Input: part model. Units: mm. Frame: model coordinates. A direction names the side the tool comes from. Round coordinates to 2 decimals unless told otherwise and drop trailing zeros. Loops run counter-clockwise (first coordinate to the right, second up) from the corner with the lowest first, then second, coordinate; pieces in that order, holes last. Notation, with made-up numbers: (57.25, -35) -> (102.25, -35) arc R19 cw to (102.25, -31) -> close; hole circle Ø4 at (56, -15.5). An arc over 180 degrees is marked (long way). Answer in a Markdown table with one row per item. Add a question column.
Q1. Section A-A, the plane z = 61. Output: boundary loops of the cut face in (x, y), and give its area (3 significant figures).
Q2. Section D-D, the plane x = -3. Output: boundary loops of the cut face in (y, z).
Q3. Section C-C, the plane x = -71.5. Output: boundary loops of the cut face in (y, z), and give its area (3 significant figures).
Q4. Ray query, L1, parallel to X at y = 23, z = -43; L2, parallel to X at y = 9, z = 58; L3, parallel to Z at x = 46, y = 36. Return the intervals inside material, ascending. Write a range as from..to.
Q5. Mould query, pull axis X, two halves, no side actions, for faces 1 (the face through (1, 40, -41)), 2 (the face through (-25, 20, -140)), 3 (the face through (-18.714, 20, 69)). Classes: pulls with the +X half, pulls with the -X half, needs draft (parallel to the pull), parting line crosses it, or undercut.
Q6. Reachability of faces 4 (the face through (-76, 20, 20)), 5 (the face through (45.714, 20, 41)), 6 (the face through (76, 20, 20)), 7 (the face through (56, 20, -120)) from +Z, -Z, +X, -X, +Y, -Y: full face, straight path, thin tool, end or side. Return the list, or none.
Q7. Pin query (flat end, axial travel): pin 1 (10 mm diameter, centred on y = 36, z = 23, fed in from +X); pin 2 (12 mm diameter, centred on y = 11.5, z = -133.5, fed in from -X); pin 3 (12 mm diameter, centred on y = 19.5, z = 86.5, fed in from -X); pin 4 (10 mm diameter, centred on x = 56.5, y = 18, fed in from +Z). Return the tip coordinate at first contact, or that it passes through.
Q8. Section B-B, the plane y = 10.5. Output: boundary loops of the cut face in (x, z), and give its area (3 significant figures).
Autodesk Inventor part; units mm, degrees
ref_plane "YZ Plane" through (0, 0, 0) normal (1, 0, 0) x (0, 1, 0)
ref_plane "XZ Plane" through (0, 0, 0) normal (0, 1, 0) x (-1, 0, 0)
ref_plane "XY Plane" through (0, 0, 0) normal (0, 0, 1) x (1, 0, 0)
sketch "スケッチ1" plane through (0, 0, 0) normal (0, 1, 0) x (-1, 0, 0)
  line L0 (45.7143, 140) -> (25.7143, 140)
  line L1 (25.7143, 140) -> (25.7143, 0)
  line L2 (25.7143, 0) -> (45.7143, 0)
  line L3 (45.7143, 0) -> (45.7143, 140)
  line L4 (45.7143, 0) -> (0, 0)
  line L5 (0, 0) -> (0, -120)
  line L6 (0, -120) -> (45.7143, -120)
  line L7 (45.7143, -120) -> (45.7143, 0)
  line L8 (25, -120) -> (0, -120)
  line L9 (0, -120) -> (0, -160)
  line L10 (0, -160) -> (25, -160)
  line L11 (25, -160) -> (25, -120)
  line L12 (45.7143, -120) -> (65.7143, -120)
  line L13 (65.7143, -120) -> (65.7143, -60)
  line L14 (65.7143, -60) -> (45.7143, -60)
  line L15 (45.7143, -60) -> (45.7143, -120)
  line L16 (65.7143, -120) -> (85.7143, -120)
  line L17 (85.7143, -120) -> (85.7143, 20)
  line L18 (85.7143, 20) -> (65.7143, 20)
  line L19 (65.7143, 20) -> (65.7143, -120)
  line L20 (0, -220) -> (0, 200)
  line L21 (102.8571, 0) -> (-17.1429, 0)
  line L22 (25.7143, 0) -> (25.7143, 140)
  line L23 (25.7143, 0) -> (18.7143, 0)
  line L24 (18.7143, 0) -> (18.7143, 140)
  line L25 (18.7143, 140) -> (25.7143, 140)
  line L26 (25.7143, 140) -> (25.7143, 0)
  point P0 (0, 0)
  point P1 (65.7143, 0)
  point P2 (25.7143, 0)
  point P3 (18.7143, 0)
  dimension "d0" = 40
  dimension "d2" = 300
  dimension "d3" = 140
  dimension "d4" = 85.7143
  dimension "d5" = 20
  dimension "d6" = 20
  dimension "d7" = 25
  dimension "d10" = 60
  dimension "d11" = 7
extrude "押し出し1" add sketch "スケッチ1" along normal blind 40 contours L3 L2 L1 L0 | L1 L4 L24 L25 | L7 L6 L5 L4 L2 | L14 L13 L12 L7 | L21 L17 L16 L13 L19 | L19 L18 L17 L21 | L11 L10 L9 L6
mirror "ミラー1" about plane through (0, 0, 0) normal (1, 0, 0)
properties part number "human_model"
Answer block:
| question | item | result |
|---|---|---|
| 1 | outline | (-45.71, 0) -> (-18.71, 0) -> (-18.71, 40) -> (-45.71, 40) -> close; (18.71, 0) -> (45.71, 0) -> (45.71, 40) -> (18.71, 40) -> close |
| 1 | area | 2,160 mm^2 |
| 2 | outline | (0, -160) -> (40, -160) -> (40, 0) -> (0, 0) -> close |
| 3 | outline | (0, -120) -> (40, -120) -> (40, 20) -> (0, 20) -> close |
| 3 | area | 5,600 mm^2 |
| 4 | L1 | -85.71..-65.71, -45.71..45.71, 65.71..85.71 |
| 4 | L2 | -45.71..-18.71, 18.71..45.71 |
| 4 | L3 | -120..-60 |
| 5 | face 1 | needs draft |
| 5 | face 2 | pulls with the -X half |
| 5 | face 3 | undercut |
| 6 | face 4 | +Z, -X, +Y, -Y |
| 6 | face 5 | +Z, +Y, -Y |
| 6 | face 6 | +Z, +X, +Y, -Y |
| 6 | face 7 | -Z, +X, +Y, -Y |
| 7 | pin 1 | x = 85.71 |
| 7 | pin 2 | x = -25 |
| 7 | pin 3 | x = -45.71 |
| 7 | pin 4 | z = -60 |
| 8 | outline | (-85.71, -120) -> (-25, -120) -> (-25, -160) -> (25, -160) -> (25, -120) -> (85.71, -120) -> (85.71, 20) -> (65.71, 20) -> (65.71, -60) -> (45.71, -60) -> (45.71, 140) -> (18.71, 140) -> (18.71, 0) -> (-18.71, 0) -> (-18.71, 140) -> (-45.71, 140) -> (-45.71, -60) -> (-65.71, -60) -> (-65.71, 20) -> (-85.71, 20) -> close |
| 8 | area | 28,500 mm^2 |
